Read the model definition and answer for the solid it produces. Units are mm, in the model's axes. Face numbers are marked on the shaded views. A direction names the side the tool comes from. Coordinates: 2 decimals unless noted, no trailing zeros. Loops run counter-clockwise (first coordinate to the right, second up) from the corner with the lowest first, then second, coordinate; pieces in that order, holes last. Notation, with made-up numbers: (9.5, 61.25) -> (42.5, 61.25) arc R28 ccw to (42.5, 97.25) -> close; hole circle Ø9 at (-37.5, 54). An arc over 180 degrees is marked (long way). Answer as CSV lines item,"result".
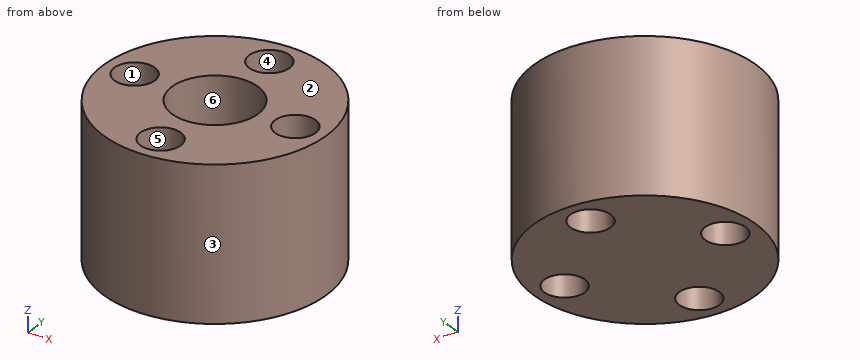
```python
from build123d import *

# Parameters (mm, degrees)
SKETCH1_R           = 11
BOSS_EXTRUDE1_DEPTH = 15
SKETCH3_R           = 2
CUT_EXTRUDE1_DEPTH  = 15
SKETCH4_R           = 4.25
CUT_EXTRUDE2_DEPTH  = 10


with BuildPart() as part:
    # Sketch1 → Boss-Extrude1 (new body)
    with BuildSketch(Plane.XY):
        Circle(SKETCH1_R)
    extrude(amount=BOSS_EXTRUDE1_DEPTH)

    # Sketch3 → Cut-Extrude1 (cut)
    with BuildSketch(Plane.XY.offset(15)):
        with Locations((-8, 0)):
            Circle(SKETCH3_R)
        with Locations((0, 8)):
            Circle(SKETCH3_R)
        with Locations((8, 0)):
            Circle(SKETCH3_R)
        with Locations((0, -8)):
            Circle(SKETCH3_R)
    extrude(amount=-CUT_EXTRUDE1_DEPTH, mode=Mode.SUBTRACT)

    # Sketch4 → Cut-Extrude2 (cut)
    with BuildSketch(Plane.XY.offset(15)):
        Circle(SKETCH4_R)
    extrude(amount=-CUT_EXTRUDE2_DEPTH, mode=Mode.SUBTRACT)


solid = part.part
```
Q1. A cutting plane is placed at C-C, the plane z = 9.5. Write down the section's boundary in (x, y), and give its area (3 significant figures).
Results:
outline,"circle Ø22 at (0, 0); hole circle Ø4 at (-8, 0); hole circle Ø8.5 at (0, 0); hole circle Ø4 at (0, -8); hole circle Ø4 at (0, 8); hole circle Ø4 at (8, 0)"
area,"273 mm²"
Q2. A cutting plane is placed at A-A, the plane x = 0. Write down the section's boundary in (y, z), and give its area (3 significant figures).
Results:
outline,"(-11, 0) -> (-10, 0) -> (-10, 15) -> (-11, 15) -> close; (-6, 0) -> (6, 0) -> (6, 15) -> (4.25, 15) -> (4.25, 5) -> (-4.25, 5) -> (-4.25, 15) -> (-6, 15) -> close; (10, 0) -> (11, 0) -> (11, 15) -> (10, 15) -> close"
area,"125 mm²"
Q3. For a pull along X with two mould halves and no side action, classify the marked faces 1, 2, 3 and 4 as pulls with the +X half, pulls with the -X half, needs draft (parallel to the pull), parting line crosses it, or undercut.
Results:
face 1,"undercut"
face 2,"needs draft"
face 3,"parting line crosses it"
face 4,"undercut"
Q4. Find the intervals of material crossed by probe 1 along Y at (x, z) = (0, 9.75); probe 2 along Y at (x, z) = (8, 12); probe 3 along X at (y, z) = (-1.25, 11), in increasing order. Write a range as [from, to].
Results:
probe 1,"y = [-11, -10], [-6, -4.25], [4.25, 6], [10, 11]"
probe 2,"y = [-7.55, -2], [2, 7.55]"
probe 3,"x = [-10.93, -9.56], [-6.44, -4.06], [4.06, 6.44], [9.56, 10.93]"
Q5. A cutting plane is placed at D-D, the plane y = -7.5. Write down the section's boundary in (x, z).
Results:
outline,"(-8.05, 0) -> (-1.94, 0) -> (-1.94, 15) -> (-8.05, 15) -> close; (1.94, 0) -> (8.05, 0) -> (8.05, 15) -> (1.94, 15) -> close"
Q6. For the marked faces 5 and 6, determine the directions among +Z, -Z, +X, -X, +Y, -Y from which every point of the face is accessible in a straight line to the end or side of a thin tool.
Results:
face 5,"+Z, -Z"
face 6,"+Z"
Q7. Given pin 1 Ø8 at (x, z) = (8, 10) entering from +Y; pin 2 Ø5 at (x, z) = (5, 11.5) entering from +Y; pin 3 Ø3 at (y, z) = (3.5, 1.5) entering from +X, each flat-ended and moving along its own axis, determine where each tip first touches the part or whether it passes through.
Results:
pin 1,"stops at y = 10.25"
pin 2,"stops at y = 10.71"
pin 3,"stops at x = 10.82"
